```python
from build123d import *

# Parameters (mm, degrees)
SKETCH_1_R               = 32
EXTRUDE_1_DEPTH          = 5
CUT_EXTRUDE_1_REACH      = 47.53
SKETCH_3_R               = 9
PATTERN_CIRCULAR_1_COUNT = 10
PATTERN_CIRCULAR_2_COUNT = 6


with BuildPart() as part:
    # Sketch 1 → Extrude 1 (new body)
    with BuildSketch(Plane.XY):
        Circle(SKETCH_1_R)
    extrude(amount=EXTRUDE_1_DEPTH)

    # Sketch 3 → Cut-Extrude 1 (cut, up to next)
    with BuildSketch(Plane(origin=(0, 0, 0), x_dir=(-1, 0, 0), z_dir=(0, 0, -1)), mode=Mode.PRIVATE) as cut_extrude_1_sk1:
        Circle(SKETCH_3_R)
    cut_extrude_1_tool1 = extrude(cut_extrude_1_sk1.sketch, amount=-CUT_EXTRUDE_1_REACH, mode=Mode.PRIVATE) & part.part
    add(cut_extrude_1_tool1.solids().sort_by_distance((0, 0, 0))[0], mode=Mode.SUBTRACT)

    # Sketch 5 → Hole Wizard 1 (revolve, cut)
    with BuildSketch(Plane(origin=(0, 27.5, 0), x_dir=(0, 1, 0), z_dir=(1, 0, 0))):
        Polygon((0, 0), (0, 8.351936393), (2.25, 7), (2.25, 0.5), (5, 0.5), (5, 0), align=None)
    hole_wizard_1 = revolve(axis=Axis((0, 27.5, -6.35), (0, 0, 1)), mode=Mode.SUBTRACT)

    # Pattern Circular 1: Hole Wizard 1 ×10 about axis
    pattern_circular_1_axis = Axis((0, 0, 0), (0, 0, 1))
    for i in range(1, PATTERN_CIRCULAR_1_COUNT):
        add(hole_wizard_1.rotate(pattern_circular_1_axis, i * 360 / PATTERN_CIRCULAR_1_COUNT), mode=Mode.SUBTRACT)

    # Sketch 10 → Hole Wizard 2 (revolve, cut)
    with BuildSketch(Plane(origin=(5.372375851, 16.654956551, 0), x_dir=(0, 1, 0), z_dir=(1, 0, 0))):
        Polygon((0, 0), (0, 7.951936393), (2.25, 6.6), (2.25, 0.5), (5, 0.5), (5, 0), align=None)
    hole_wizard_2 = revolve(axis=Axis((5.372375851, 16.654956551, -6.35), (0, 0, 1)), mode=Mode.SUBTRACT)

    # Pattern Circular 2: Hole Wizard 2 ×6 about axis
    pattern_circular_2_axis = Axis((0, 0, 0), (0, 0, 1))
    for i in range(1, PATTERN_CIRCULAR_2_COUNT):
        add(hole_wizard_2.rotate(pattern_circular_2_axis, i * 360 / PATTERN_CIRCULAR_2_COUNT), mode=Mode.SUBTRACT)


solid = part.part
```
Verification items for the finished model (mm, model axes). A direction names the side the tool comes from. Coordinates: 2 decimals unless noted, no trailing zeros. Loops run counter-clockwise (first coordinate to the right, second up) from the corner with the lowest first, then second, coordinate; pieces in that order, holes last. Notation, with made-up numbers: (29.25, -25) -> (35.25, -25) arc R25 ccw to (35.25, 10) -> close; hole circle Ø9 at (67.25, 42.5). An arc over 180 degrees is marked (long way). Answer in a Markdown table with one row per item. Add a question column.
1. Access from +Z, -Z, +X, -X, +Y, -Y to the whole of each face (thin tool, end or side, straight path). Record for faces 1 (the face through (0.186, -22.503, 0.246)), 2 (the face through (17.209, 5.923, 2.718)).
2. Section check B-B, the plane z = 2.9. Give the number of separate pieces and of enclosed holes in the cut face, then the cut area to 3 significant figures.
3. Section check A-A, the plane y = 10. Enter the section's corners in (x, z) (3 decimals), then the cut area to 3 significant figures.
4. Draft check along Y on faces 3 (the face through (7, -7, 0)), 4 (the face through (-28.404, 8.518, 2.719)). Enter one of: +Y half, -Y half, draft (parallel to the pull), parting line (faces both ways), or undercut.
5. Depth check by flat-ended pin: P1, Ø2.5, axis at x = -11.74, y = 12.98, coming from the -Z side; P2, Ø9, axis at x = -17.11, y = -3.67, coming from the -Z side; P3, Ø1.5, axis at x = -24.5, z = 3, coming from the -Y side; P4, Ø2, axis at x = -5, z = 4, coming from the +Y side. Enter the tip coordinate at first touch or a pass-through.
6. Material ranges on probe 1 along Y at (x, z) = (-6, 4.4); probe 2 along Y at (x, z) = (-17, 4.45); probe 3 along X at (y, z) = (3, 4.45), recorded low to high. Write a range as [from, to].
7. Section check C-C, the plane y = 0. Enter the section's corners in (x, z), then the cut area to 3 significant figures.
Derived:
| question | item | result |
|---|---|---|
| 1 | face 1 | -Z |
| 1 | face 2 | +Z, -Z |
| 2 | separate pieces | 1 |
| 2 | enclosed holes | 17 |
| 2 | area | 2,710 mm² |
| 3 | outline | (-30.397, 0.5) -> (-27.829, 0.5) -> (-27.829, 5) -> (-30.397, 5) -> close; (-24.479, 0.5) -> (-21.385, 0.5) -> (-21.385, 0) -> (-15.752, 0) -> (-15.752, 0.5) -> (-7.723, 0.5) -> (-7.723, 0) -> (21.385, 0) -> (21.385, 0.5) -> (24.479, 0.5) -> (24.479, 5) -> (-24.479, 5) -> close; (27.829, 0.5) -> (30.397, 0.5) -> (30.397, 5) -> (27.829, 5) -> close |
| 3 | area | 261 mm² |
| 4 | face 3 | draft |
| 4 | face 4 | undercut |
| 5 | P1 | passes through |
| 5 | P2 | stops at z = 0.5 |
| 5 | P3 | stops at y = -21.45 |
| 5 | P4 | stops at y = 31.75 |
| 6 | probe 1 | y = [-31.43, -18.82], [-14.49, -6.71], [6.71, 31.43] |
| 6 | probe 2 | y = [-27.11, -24.34], [-20.16, -5.92], [-1.43, 20.16], [24.34, 27.11] |
| 6 | probe 3 | x = [-31.86, -8.49], [8.49, 14.96], [19.26, 31.86] |
| 7 | outline | (-32, 0) -> (-20.5, 0) -> (-20.5, 0.5) -> (-13.72, 0.5) -> (-13.72, 0) -> (-9, 0) -> (-9, 5) -> (-32, 5) -> close; (9, 0) -> (13.72, 0) -> (13.72, 0.5) -> (20.5, 0.5) -> (20.5, 0) -> (32, 0) -> (32, 5) -> (9, 5) -> close |
| 7 | area | 223 mm² |
